Verification items for the finished model (mm, model axes). Face numbers are marked on the shaded views. A direction names the side the tool comes from. Give positions to 0.01 mm unless a question says otherwise; leave off trailing zeros. Loops run counter-clockwise (first coordinate to the right, second up) from the corner with the lowest first, then second, coordinate; pieces in that order, holes last. Notation, with made-up numbers: (-13, -23.5) - (7, -23.5) arc R17 ccw to (7, -11.5) - close; hole circle Ø7 at (18.25, 5.25). An arc over 180 degrees is marked (long way). Answer in a Markdown table with one row per item.
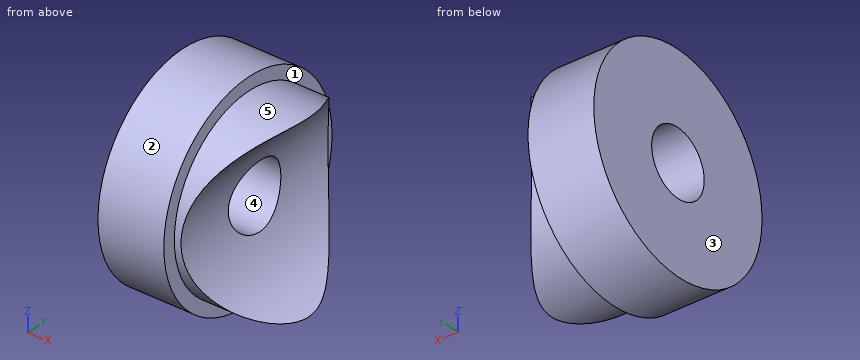
```python
from build123d import *

# Parameters (mm, degrees)
SKETCH1_R               = 8
BOSS_EXTRUDE1_DEPTH     = 5
SKETCH2_R               = 7
BOSS_EXTRUDE2_DEPTH     = 5
CUT_EXTRUDE1_DEPTH      = 16.099668871
CUT_EXTRUDE1_DEPTH_BACK = 15
SKETCH3_R               = 8
SKETCH4_R               = 2.5
CUT_EXTRUDE2_DEPTH      = 15


with BuildPart() as part:
    # Sketch1 → Boss-Extrude1 (new body)
    with BuildSketch(Plane(origin=(0, 0, 0), x_dir=(0, 0, -1), z_dir=(1, 0, 0))):
        Circle(SKETCH1_R)
    extrude(amount=BOSS_EXTRUDE1_DEPTH)

    # Sketch2 → Boss-Extrude2 (add)
    with BuildSketch(Plane(origin=(5, 0, 0), x_dir=(0, 0, -1), z_dir=(1, 0, 0))):
        Circle(SKETCH2_R)
    extrude(amount=BOSS_EXTRUDE2_DEPTH)

    # Sketch3 → Cut-Extrude1 (cut, two sides: drawn at the far end of the back side and taken through both)
    with BuildSketch(Plane(origin=(0, 0, 0), x_dir=(1, 0, 0), z_dir=(0, 1, 0)).offset(-CUT_EXTRUDE1_DEPTH_BACK)):
        with Locations((13.5, 0)):
            Circle(SKETCH3_R)
    extrude(amount=CUT_EXTRUDE1_DEPTH + CUT_EXTRUDE1_DEPTH_BACK, mode=Mode.SUBTRACT)

    # Sketch4 → Cut-Extrude2 (cut)
    with BuildSketch(Plane.ZY):
        Circle(SKETCH4_R)
    extrude(amount=-CUT_EXTRUDE2_DEPTH, mode=Mode.SUBTRACT)


solid = part.part
```
Q1. Sectioned sample at B-B (z = 0). Record the cut outline in (x, y).
Completed:
| item | result |
|---|---|
| outline | (0, -8) - (5, -8) - (5, -7) - (5.5, -7) - (5.5, -2.5) - (0, -2.5) - close; (0, 2.5) - (5.5, 2.5) - (5.5, 7) - (5, 7) - (5, 8) - (0, 8) - close |
Q2. Sectioned sample at A-A (y = 0). Record the cut outline in (x, z), and give its area (3 significant figures).
Completed:
| item | result |
|---|---|
| outline | (0, -8) - (5, -8) - (5, -7) - (9.63, -7) arc R8 cw to (5.9, -2.5) - (0, -2.5) - close; (0, 2.5) - (5.9, 2.5) arc R8 cw to (9.63, 7) - (5, 7) - (5, 8) - (0, 8) - close |
| area | 75.5 mm^2 |
Q3. Draft check along Y on the marked faces 3, 4 and 5. Enter one of: +Y half, -Y half, draft (parallel to the pull), parting line (faces both ways), or undercut.
Completed:
| item | result |
|---|---|
| face 3 | draft |
| face 4 | undercut |
| face 5 | parting line |
Q4. Tool access check on the marked faces 1 and 2. Record the directions out of +Z, -Z, +X, -X, +Y, -Y that give a thin tool (end or side, any length) a straight path to the whole face; none if there is none.
Completed:
| item | result |
|---|---|
| face 1 | +X |
| face 2 | +X, -X |
Q5. Thickness scan on line 1 (Y direction, x = 1.3, z = 0); line 2 (X direction, y = 5.5, z = 5.5); line 3 (Z direction, x = 6.5, y = 0.75). Record the ranges inside material, lowest first.
Completed:
| item | result |
|---|---|
| line 1 | -8 to -2.5, 2.5 to 8 |
| line 2 | 0 to 5 |
| line 3 | -6.96 to -3.87, 3.87 to 6.96 |
Q6. Sectioned sample at C-C (x = 2.5). Record the cut outline in (y, z), and give its area (3 significant figures).
Completed:
| item | result |
|---|---|
| outline | circle Ø16 at (0, 0); hole circle Ø5 at (0, 0) |
| area | 181 mm^2 |
Q7. Sectioned sample at D-D (z = 3.75). Record the cut outline in (x, y).
Completed:
| item | result |
|---|---|
| outline | (0, -7.07) - (5, -7.07) - (5, -5.91) - (6.43, -5.91) - (6.43, 5.91) - (5, 5.91) - (5, 7.07) - (0, 7.07) - close |
Q8. Go/stop test with flat-tipped pins: P1, Ø2, axis at x = 3.5, y = 5, coming from the -Z side; P2, Ø8, axis at y = 4, z = -6, coming from the +X side; P3, Ø5, axis at x = 8, z = 3, coming from the -Y side. Record where each tip stops, or that it passes through.
Completed:
| item | result |
|---|---|
| P1 | z = -6.93 |
| P2 | x = 9.62 |
| P3 | y = -6.73 |
